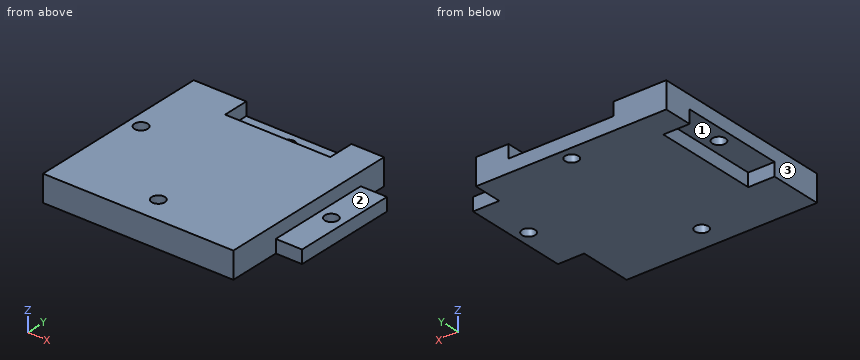
Autodesk Inventor part; units mm, degrees
ref_plane "YZ Plane" through (0, 0, 0) normal (1, 0, 0) x (0, 1, 0)
ref_plane "XZ Plane" through (0, 0, 0) normal (0, 1, 0) x (-1, 0, 0)
ref_plane "XY Plane" through (0, 0, 0) normal (0, 0, 1) x (1, 0, 0)
sketch "Sketch1" plane through (0, 0, 0) normal (0, 0, 1) x (1, 0, 0)
  line L0 (0, 0) -> (72.4, 0)
  line L1 (72.4, 0) -> (72.4, 71)
  line L2 (72.4, 71) -> (0, 71)
  line L3 (0, 71) -> (0, 0)
  dimension "d0" = 72.4
  dimension "d1" = 71
extrude "Extrusion1" add sketch "Sketch1" along normal blind 10
sketch "Sketch2" plane through (0, 0, 10) normal (0, 0, 1) x (1, 0, 0)
  line L0 (72.4, 0) -> (72.4, 71)
  line L1 (72.4, 20) -> (82.4, 20)
  line L2 (82.4, 20) -> (82.4, 60)
  line L3 (82.4, 60) -> (72.4, 60)
  line L4 (72.4, 60) -> (72.4, 20)
  line L5 (72.4, 71) -> (0, 71)
  circle A0 centre (77.4, 40) radius 2.5
  line L6 (0, 0) -> (72.4, 0)
  point P0 (82.4, 40)
  point P1 (77.4, 60)
  dimension "d4" = 10
  dimension "d5" = 40
  dimension "d7" = 5
  dimension "d22" = 20
extrude "Extrusion2" add sketch "Sketch2" against normal blind 10
sketch "Sketch3" plane through (0, 0, 10) normal (0, 0, 1) x (1, 0, 0)
  line L0 (72.4, 60) -> (82.4, 60)
  line L1 (72.4, 20) -> (82.4, 20)
  line L2 (82.4, 60) -> (72.4, 60)
  line L3 (72.4, 60) -> (72.4, 20)
  line L4 (72.4, 20) -> (82.4, 20)
  line L5 (82.4, 20) -> (82.4, 60)
  point P0 (0, 0)
extrude "Extrusion3" cut sketch "Sketch3" against normal blind 5
sketch "Sketch4" plane through (0, 0, 0) normal (0, 0, -1) x (-1, 0, 0)
  line L0 (0, 71) -> (0, 0)
  line L1 (0, 60) -> (-10, 60)
  line L2 (-10, 60) -> (-10, 20)
  line L3 (-10, 20) -> (0, 20)
  line L4 (0, 20) -> (0, 60)
  point P0 (-72.4, 60)
  dimension "d15" = 10
  dimension "d16" = 40
extrude "Extrusion4" cut sketch "Sketch4" against normal blind 5
sketch "Sketch5" plane through (0, 0, 5) normal (0, 0, -1) x (-1, 0, 0)
  circle A0 centre (-5, 40) radius 2.5
  line L0 (0, 60) -> (0, 20)
  line L1 (-10, 60) -> (0, 60)
  point P0 (0, 0)
  point P1 (0, 40)
  point P2 (-5, 60)
  dimension "d19" = 5
extrude "Extrusion5" cut sketch "Sketch5" against normal through all
sketch "Sketch6" plane through (0, 0, 10) normal (0, 0, 1) x (1, 0, 0)
  line L0 (72.4, 71) -> (0, 71)
  line L1 (60, 71) -> (20, 71)
  line L2 (20, 71) -> (20, 61)
  line L3 (20, 61) -> (60, 61)
  line L4 (60, 61) -> (60, 71)
  line L5 (0, 71) -> (0, 0)
  dimension "d23" = 40
  dimension "d24" = 10
  dimension "d25" = 20
extrude "Extrusion6" cut sketch "Sketch6" against normal blind 5
sketch "Sketch7" plane through (0, 0, 5) normal (0, 0, 1) x (1, 0, 0)
  circle A0 centre (40, 66) radius 2.5
  line L0 (60, 61) -> (20, 61)
  line L1 (20, 61) -> (20, 71)
  point P0 (0, 0)
  point P1 (40, 61)
  point P2 (20, 66)
  dimension "d28" = 5
extrude "Extrusion7" cut sketch "Sketch7" against normal through all
sketch "Sketch8" plane through (0, 0, 10) normal (0, 0, 1) x (1, 0, 0)
  circle A0 centre (36.2, 9.5) radius 2.5
  line L0 (0, 0) -> (72.4, 0)
  point P0 (36.2, 0)
  dimension "d31" = 5
  dimension "d32" = 9.5
extrude "Extrusion8" cut sketch "Sketch8" against normal through all
properties part number "SP002" material "ABS Plastic"
Design review of the part built by this model. Coordinates are the model's own, in mm. Face numbers are marked on the shaded views. A direction names the side the tool comes from. Coordinates: 2 decimals unless noted, no trailing zeros. Loops run counter-clockwise (first coordinate to the right, second up) from the corner with the lowest first, then second, coordinate; pieces in that order, holes last.
Item 1: Add section B-B (y = 40). Write out the cut boundary in (x, z), and give its area (3 significant figures).
Completed:
outline: (0, 5) - (2.5, 5) - (2.5, 10) - (0, 10) - close; (7.5, 5) - (10, 5) - (10, 0) - (74.9, 0) - (74.9, 5) - (72.4, 5) - (72.4, 10) - (7.5, 10) - close; (79.9, 0) - (82.4, 0) - (82.4, 5) - (79.9, 5) - close
area: 674 mm2
Item 2: Add section C-C (x = 77.4). Write out the cut boundary in (y, z).
Completed:
outline: (20, 0) - (37.5, 0) - (37.5, 5) - (20, 5) - close; (42.5, 0) - (60, 0) - (60, 5) - (42.5, 5) - close
Item 3: Clearance check with flat-ended pins moving along their axes: pin 1 (2.5 mm diameter, centred on x = 38.5, z = 7, fed in from +Y); pin 2 (3 mm diameter, centred on x = 6.5, y = 39.5, fed in from -Z); pin 3 (4.5 mm diameter, centred on x = 77.4, y = 40, fed in from -Z); pin 4 (4 mm diameter, centred on x = 78.5, z = 3.5, fed in from +Y). State where each tip first meets the part, or that it passes through.
Completed:
pin 1: stops at y = 61
pin 2: stops at z = 5
pin 3: passes through
pin 4: stops at y = 60
Item 4: For the marked faces 1, 2 and 3, list the 3-axis set-ups (+Z, -Z, +X, -X, +Y, -Y) from which the entire face can be reached by the end or side of a thin tool; tool diameter is ignored.
Completed:
face 1: -Z, -X
face 2: +Z, +X, +Y, -Y
face 3: +Z, -Z, -X, +Y, -Y
Item 5: Add section A-A (y = 9.5). Write out the cut boundary in (x, z), and give its area (3 significant figures).
Completed:
outline: (0, 0) - (33.7, 0) - (33.7, 10) - (0, 10) - close; (38.7, 0) - (72.4, 0) - (72.4, 10) - (38.7, 10) - close
area: 674 mm2
Item 6: Add section D-D (z = 3). Write out the cut boundary in (x, y).
Completed:
outline: (0, 0) - (72.4, 0) - (72.4, 20) - (82.4, 20) - (82.4, 60) - (72.4, 60) - (72.4, 71) - (0, 71) - (0, 60) - (10, 60) - (10, 20) - (0, 20) - close; hole circle Ø5 at (36.2, 9.5); hole circle Ø5 at (40, 66); hole circle Ø5 at (77.4, 40)
Item 7: Wall thickness on L1, parallel to Y at x = 40, z = 1.9; L2, parallel to Y at x = 5, z = 6.1; L3, parallel to Y at x = 47, z = 5.5: over which ranges is each line inside the solid? List them lowest first.
Completed:
L1: y = 0 to 63.5, 68.5 to 71
L2: y = 0 to 37.5, 42.5 to 71
L3: y = 0 to 61
